from build123d import *

# Parameters (mm, degrees)
BOSS_EXTRUDE1_DEPTH = 50
BOSS_EXTRUDE2_START = 50
BOSS_EXTRUDE2_DEPTH = 10
SKETCH2_R           = 15
SKETCH2_R_2         = 12
BOSS_EXTRUDE3_DEPTH = 5
BOSS_EXTRUDE4_DEPTH = 25
FILLET1_R           = 2


with BuildPart() as part:
    # Sketch1 → Boss-Extrude1 (new body)
    with BuildSketch(Plane.XY):
        Polygon((10, 10), (0, 0), (100, 0), (90, 10), (90, 20), (45, 20), (10, 20), align=None)
    extrude(amount=BOSS_EXTRUDE1_DEPTH)

    # Sketch1<4> → Boss-Extrude2 (add)
    with BuildSketch(Plane.XY.offset(BOSS_EXTRUDE2_START)):
        Polygon((10, 45), (10, 20), (45, 20), (20, 45), align=None)
    extrude(amount=-BOSS_EXTRUDE2_DEPTH)

    # Sketch2 → Boss-Extrude3 (add)
    with BuildSketch(Plane(origin=(0, 20, 0), x_dir=(1, 0, 0), z_dir=(0, 1, 0))):
        with Locations((65, -25)):
            Circle(SKETCH2_R)
        with Locations(Location((65, -25, 0), (0, 0, 180))):
            Circle(SKETCH2_R_2, mode=Mode.SUBTRACT)
    extrude(amount=BOSS_EXTRUDE3_DEPTH)

    # Sketch2<3> → Boss-Extrude4 (add)
    with BuildSketch(Plane(origin=(0, 20, 0), x_dir=(1, 0, 0), z_dir=(0, 1, 0))):
        Polygon((10, -40), (20, -40), (20, -10), (50, -10), (50, 0), (10, 0), align=None)
    extrude(amount=BOSS_EXTRUDE4_DEPTH)

    # Fillet1
    fillet1_edges = [part.edges().sort_by_distance(p)[0] for p in [
        (50, 20, 25),
    ]]
    fillet(fillet1_edges, radius=FILLET1_R)


solid = part.part
The model under review builds one solid part; all positions refer to its coordinate system, in mm. A direction names the side the tool comes from. Give positions to 0.01 mm unless a question says otherwise; leave off trailing zeros. Order: outer loops, then holes, each group sorted by start corner. A loop starts at its lowest first (then second) coordinate and runs counter-clockwise, first axis right, second up. Notation, with made-up numbers: M -29,58 L 19,58 A25 cw 19,94 Z; hole C 1,11 d4. An arc over 180 degrees is marked long. Use one line per item in the form item = value. Start each with the question number.
Item 1: We need section D-D on z = 25. Give the boundary of the cut face in (x, y), plus the area to 3 significant figures.
Item 2: We need section C-C on x = 65. Give the boundary of the cut face in (y, z).
Item 3: The part is to be moulded in two halves that separate along X. For faces 6 (the flat face through (58, 25, 15)), 7 (the flat face through (95, 5, 25)), 8 (the cylindrical face through (53, 23, 34)), 9 (the flat face through (65, 20, 25)), say which applies: pulls with the +X half, pulls with the -X half, needs draft (parallel to the pull), parting line crosses it, or undercut.
Item 4: For faces 1 (the flat face through (10, 27, 25)), 2 (the flat face through (90, 15, 25)), 3 (the flat face through (49, 0, 25)), 4 (the flat face through (38, 13, 50)), 5 (the flat face through (35, 32, 10)), list the 3-axis set-ups (+Z, -Z, +X, -X, +Y, -Y) from which the entire face can be reached by the end or side of a thin tool; tool diameter is ignored.
Item 5: Insertion check: pin 1 Ø6 at (y, z) = (11.5, 18) entering from -X; pin 2 Ø2 at (y, z) = (9, 7.5) entering from +X; pin 3 Ø2 at (y, z) = (12.5, 7) entering from -X; pin 4 Ø4 at (x, z) = (11, 11.5) entering from -Y. Each pin has a flat end and moves straight along its axis. Give the tip position at first contact, or say it passes through.
Item 6: To check wall thickness, follow line 1 along X through (y, z) = (24.5, 30.5); line 2 along Z through (x, y) = (31, 23); line 3 along Z through (x, y) = (65, 23.5). State the ranges of each line that lie inside material, in increasing order. Write a range as from..to.
Item 7: We need section B-B on y = 32. Give the boundary of the cut face in (x, z), plus the area to 3 significant figures.
Item 8: We need section A-A on z = 45.5. Give the boundary of the cut face in (x, y).
Completed:
q1.outline = M 0,0 L 100,0 L 90,10 L 90,20 L 82,20 A2 cw 80,22 L 80,25 L 77,25 L 77,20 L 53,20 L 53,25 L 50,25 L 50,22 A2 cw 48,20 L 20,20 L 20,45 L 10,45 L 10,10 Z
q1.area = 1,980 mm²
q2.outline = M 0,0 L 20,0 L 20,8 A2 cw 22,10 L 25,10 L 25,13 L 20,13 L 20,37 L 25,37 L 25,40 L 22,40 A2 cw 20,42 L 20,50 L 0,50 Z
q3.face_6 = needs draft
q3.face_7 = pulls with the +X half
q3.face_8 = undercut
q3.face_9 = undercut
q4.face_1 = +Z, -Z, -X, +Y
q4.face_2 = +Z, -Z, +X, +Y
q4.face_3 = +Z, -Z, +X, -X, -Y
q4.face_4 = +Z, +X, -X, +Y, -Y
q4.face_5 = +Y
q5.pin_1 = 8.5
q5.pin_2 = 92
q5.pin_3 = 10
q5.pin_4 = 0
q6.line_1 = 10..20, 51.04..54.33, 75.67..78.96
q6.line_2 = 0..10, 40..50
q6.line_3 = 10..13, 37..40
q7.outline = M 10,0 L 50,0 L 50,10 L 20,10 L 20,40 L 33,40 L 33,50 L 10,50 Z
q7.area = 930 mm²
q8.outline = M 0,0 L 100,0 L 90,10 L 90,20 L 45,20 L 20,45 L 10,45 L 10,10 Z
